Design review of the part built by this model. Coordinates are the model's own, in mm. A direction names the side the tool comes from. Coordinates: 2 decimals unless noted, no trailing zeros. Loops run counter-clockwise (first coordinate to the right, second up) from the corner with the lowest first, then second, coordinate; pieces in that order, holes last. Notation, with made-up numbers: M 11,28.5 L 40,28.5 A22 ccw 40,56.5 Z; hole C -37.5,-24.5 d6. An arc over 180 degrees is marked long. One line per item, written item: value.
```python
from build123d import *

# Parameters (mm, degrees)
CROQUIS1_R              = 7.5
SALIENTE_EXTRUIR1_DEPTH = 25
CROQUIS6_W              = 35
CROQUIS6_H              = 20
CORTAR_EXTRUIR3_DEPTH   = 103.164083709
REDONDEO3_START         = -1
REDONDEO3_DEPTH         = 27
REDONDEO3_2_DEPTH       = 25
CROQUIS7_R              = 2.5
CORTAR_EXTRUIR4_DEPTH   = 104.770178761
CROQUIS8_R              = 4.375
CORTAR_EXTRUIR5_DEPTH   = 5
CROQUIS9_R              = 2.6
CORTAR_EXTRUIR6_DEPTH   = 104.770178761
CORTAR_EXTRUIR7_DEPTH   = 4
CORTAR_EXTRUIR8_DEPTH   = 4
CORTAR_EXTRUIR9_DEPTH   = 4


with BuildPart() as part:
    # Croquis1 → Saliente-Extruir1 (new body)
    with BuildSketch(Plane(origin=(0, 0, 0), x_dir=(1, 0, 0), z_dir=(0, 1, 0))):
        with BuildLine():
            Line((88, 10.5), (0, 10.5))
            ThreePointArc((0, 10.5), (-10.5, 0), (0, -10.5))
            Line((0, -10.5), (88, -10.5))
            ThreePointArc((88, -10.5), (98.5, 0), (88, 10.5))
        make_face()
        with Locations(Location((0, 0, 0), (0, 0, 270))):
            Circle(CROQUIS1_R, mode=Mode.SUBTRACT)
        with Locations(Location((88, 0, 0), (0, 0, 270))):
            Circle(CROQUIS1_R, mode=Mode.SUBTRACT)
    extrude(amount=SALIENTE_EXTRUIR1_DEPTH)

    # Croquis6 → Cortar-Extruir3 (cut, through all)
    with BuildSketch(Plane.XZ):
        with Locations((44, 10.5)):
            Rectangle(CROQUIS6_W, CROQUIS6_H)
    extrude(amount=-CORTAR_EXTRUIR3_DEPTH, mode=Mode.SUBTRACT)

    # Redondeo3: read off the stored shape, not the designer's step
    # Redondeo3 outline → Redondeo3 (cut)
    with BuildSketch(Plane(origin=(0, 0, 0), x_dir=(1, 0, 0), z_dir=(0, 1, 0)).offset(REDONDEO3_START)):
        with BuildLine():
            Line((26.5, -10.5), (26.5, -5.5))
            ThreePointArc((26.5, -5.5), (25.035533906, -9.035533906), (21.5, -10.5))
            Line((21.5, -10.5), (26.5, -10.5))
        make_face()
        with BuildLine():
            ThreePointArc((66.5, -10.5), (62.964466094, -9.035533906), (61.5, -5.5))
            Line((61.5, -5.5), (61.5, -10.5))
            Line((61.5, -10.5), (66.5, -10.5))
        make_face()
    extrude(amount=REDONDEO3_DEPTH, mode=Mode.SUBTRACT)

    # Redondeo3 2 outline → Redondeo3 2 (add)
    with BuildSketch(Plane(origin=(0, 0, 0), x_dir=(1, 0, 0), z_dir=(0, 1, 0))):
        with BuildLine():
            Line((61.5, -0.5), (56.5, -0.5))
            ThreePointArc((56.5, -0.5), (60.035533906, -1.964466094), (61.5, -5.5))
            Line((61.5, -5.5), (61.5, -0.5))
        make_face()
        with BuildLine():
            ThreePointArc((26.5, -5.5), (27.964466094, -1.964466094), (31.5, -0.5))
            Line((31.5, -0.5), (26.5, -0.5))
            Line((26.5, -0.5), (26.5, -5.5))
        make_face()
    extrude(amount=REDONDEO3_2_DEPTH)

    # Croquis7 → Cortar-Extruir4 (cut, through all)
    with BuildSketch(Plane(origin=(0, 0, -10.5), x_dir=(-1, 0, 0), z_dir=(0, 0, -1))):
        with Locations((-35.5, 19)):
            Circle(CROQUIS7_R)
        with Locations((-35.5, 6)):
            Circle(CROQUIS7_R)
    extrude(amount=-CORTAR_EXTRUIR4_DEPTH, mode=Mode.SUBTRACT)

    # Croquis8 → Cortar-Extruir5 (cut)
    with BuildSketch(Plane(origin=(0, 0, -10.5), x_dir=(-1, 0, 0), z_dir=(0, 0, -1))):
        with Locations((-35.5, 19)):
            Circle(CROQUIS8_R)
        with Locations((-35.5, 6)):
            Circle(CROQUIS8_R)
    extrude(amount=-CORTAR_EXTRUIR5_DEPTH, mode=Mode.SUBTRACT)

    # Croquis9 → Cortar-Extruir6 (cut, through all)
    with BuildSketch(Plane(origin=(0, 0, -10.5), x_dir=(-1, 0, 0), z_dir=(0, 0, -1))):
        with Locations((-71, 12.5)):
            Circle(CROQUIS9_R)
        with Locations(Location((-17, 12.5, 0), (0, 0, 180))):
            Circle(CROQUIS9_R)
    extrude(amount=-CORTAR_EXTRUIR6_DEPTH, mode=Mode.SUBTRACT)

    # Croquis10 → Cortar-Extruir7 (cut)
    with BuildSketch(Plane.XY.offset(10.5)):
        Polygon((75.734272207, 12.5), (73.367136104, 16.6), (68.632863896, 16.6), (66.265727793, 12.5), (68.632863896, 8.4), (73.367136104, 8.4), align=None)
    extrude(amount=-CORTAR_EXTRUIR7_DEPTH, mode=Mode.SUBTRACT)

    # Croquis11 → Cortar-Extruir8 (cut)
    with BuildSketch(Plane.XY.offset(0.5)):
        Polygon((40.234272207, 6), (37.867136104, 10.1), (33.132863896, 10.1), (30.765727793, 6), (33.132863896, 1.9), (37.867136104, 1.9), align=None)
        Polygon((40.234272207, 19), (37.867136104, 23.1), (33.132863896, 23.1), (30.765727793, 19), (33.132863896, 14.9), (37.867136104, 14.9), align=None)
    extrude(amount=-CORTAR_EXTRUIR8_DEPTH, mode=Mode.SUBTRACT)

    # Croquis12 → Cortar-Extruir9 (cut)
    with BuildSketch(Plane.XY.offset(10.5)):
        Polygon((12.265727793, 12.5), (14.632863896, 8.4), (19.367136104, 8.4), (21.734272207, 12.5), (19.367136104, 16.6), (14.632863896, 16.6), align=None)
    extrude(amount=-CORTAR_EXTRUIR9_DEPTH, mode=Mode.SUBTRACT)


solid = part.part
```
(1) To check wall thickness, follow line 1 along Y through (x, z) = (35.5, -4.7); line 2 along X through (y, z) = (19.5, 0); line 3 along Y through (x, z) = (17, -6.5). State the ranges of each line that lie inside material, in increasing order. Write a range as [from, to].
Reply:
line 1: y = [0, 3.5], [8.5, 16.5], [21.5, 25]
line 2: x = [-10.5, -7.5], [7.5, 31.05], [39.95, 80.5], [95.5, 98.5]
line 3: y = [0, 9.9], [15.1, 25]
(2) Tool access review of faces 1 (the flat face through (35, 1.9, -1)), 2 (the cylindrical face through (36.07, 10.338, -8.035)), 3 (the flat face through (31.93, 16.98, -1.47)): name each direction out of +Z, -Z, +X, -X, +Y, -Y from which nothing blocks a thin tool from reaching the whole face with its end or side.
Reply:
face 1: +Z
face 2: -Z
face 3: none
(3) We need section B-B on x = 17. State the section outline as (y, z) points, then the cut area to 3 significant figures.
Reply:
outline: M 0,-10.5 L 9.9,-10.5 L 9.9,6.5 L 8.4,6.5 L 8.4,10.5 L 0,10.5 Z; M 15.1,-10.5 L 25,-10.5 L 25,10.5 L 16.6,10.5 L 16.6,6.5 L 15.1,6.5 Z
area: 404 mm2
(4) Insertion check: pin 1 (1.5 mm diameter, centred on y = 18, z = 4, fed in from +X); pin 2 (3 mm diameter, centred on y = 17.5, z = 2.5, fed in from +X); pin 3 (1.5 mm diameter, centred on y = 14, z = 4.5, fed in from -X). Each pin has a flat end and moves straight along its axis. Give the tip position at first contact, or say it passes through.
Reply:
pin 1: stops at x = 97.98
pin 2: stops at x = 98.45
pin 3: stops at x = -9.81
(5) We need section A-A on z = 8.75. State the section outline as (x, y) points, then the cut area to 3 significant figures.
Reply:
outline: M -5.8,0 L 25.3,0 L 25.3,25 L -5.8,25 Z; M 62.7,0 L 93.8,0 L 93.8,25 L 62.7,25 Z; hole M 12.27,12.5 L 14.63,8.4 L 19.37,8.4 L 21.73,12.5 L 19.37,16.6 L 14.63,16.6 Z; hole M 66.27,12.5 L 68.63,8.4 L 73.37,8.4 L 75.73,12.5 L 73.37,16.6 L 68.63,16.6 Z
area: 1,440 mm2
(6) Mouldability with a two-part tool opening along Z and no side actions: class faces 4 (the flat face through (33.6, 17.1, -5.5)), 5 (the cylindrical face through (80.68, 12.32, -1.63)), 6 (the cylindrical face through (73.6, 12.6, -2.1)) as released by +Z, released by -Z, zero draft, split by the parting line, or undercut.
Reply:
face 4: released by -Z
face 5: undercut
face 6: zero draft
